For this review, use the dimensioned drawing (mm, ordinates from the lowest corner) and the shaded views. Coordinates: 2 decimals unless noted, no trailing zeros. Loops run counter-clockwise (first coordinate to the right, second up) from the corner with the lowest first, then second, coordinate; pieces in that order, holes last. Notation, with made-up numbers: (75.5, 28) -> (84.5, 28) arc R21 cw to (84.5, 51) -> close; hole circle Ø11 at (26.5, -6.5). An arc over 180 degrees is marked (long way). One line per question, with ' | ' between items. Start each with the question number.
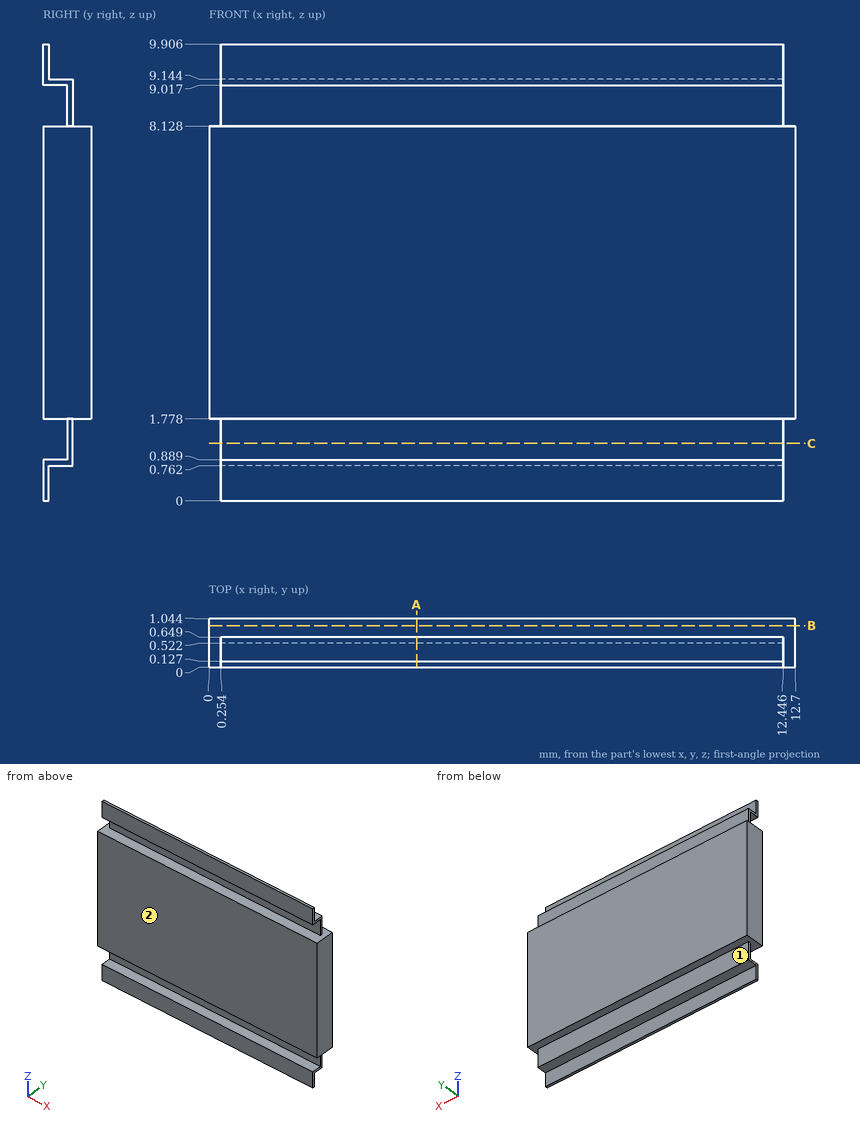
1) Consider section B-B, the plane y = 0.9. Write out the cut boundary in (x, z).
2) Consider section A-A, the plane x = 4.5. Write out the cut boundary in (y, z).
3) Insertion check: pin 1 Ø0.6 at (x, z) = (4, 0.5) entering from +Y. The pin has a flat end and moves straight along its axis. Give the tip position at first contact, or say it passes through.
4) Consider section C-C, the plane z = 1.25. Write out the cut boundary in (x, y).
5) Mouldability with a two-part tool opening along Y and no side actions: class the marked faces 1 and 2 as +Y half, -Y half, draft (parallel to the pull), parting line (faces both ways), or undercut.
6) Wall thickness on L1, parallel to Z at x = 4.75, y = 0.8: over which ranges is the line inside the solid? List them lowest first.
Filled sheet:
1) outline: (0, 1.78) -> (12.7, 1.78) -> (12.7, 8.13) -> (0, 8.13) -> close
2) outline: (0, 0) -> (0.13, 0) -> (0.13, 0.76) -> (0.65, 0.76) -> (0.65, 1.78) -> (1.04, 1.78) -> (1.04, 8.13) -> (0.65, 8.13) -> (0.65, 9.14) -> (0.13, 9.14) -> (0.13, 9.91) -> (0, 9.91) -> (0, 9.02) -> (0.52, 9.02) -> (0.52, 8.13) -> (0, 8.13) -> (0, 1.78) -> (0.52, 1.78) -> (0.52, 0.89) -> (0, 0.89) -> close
3) pin 1: y = 0.65
4) outline: (0.25, 0.52) -> (12.45, 0.52) -> (12.45, 0.65) -> (0.25, 0.65) -> close
5) face 1: +Y half | face 2: -Y half
6) L1: 1.78 to 8.13
